Verification items for the finished model (mm, model axes). A direction names the side the tool comes from. Give positions to 0.01 mm unless a question says otherwise; leave off trailing zeros. Loops run counter-clockwise (first coordinate to the right, second up) from the corner with the lowest first, then second, coordinate; pieces in that order, holes last. Notation, with made-up numbers: (-15.75, -15.75) - (23.25, -15.75) arc R16 ccw to (23.25, 4.25) - close; hole circle Ø7 at (-31, 47.5). An arc over 180 degrees is marked (long way). One line per item, written item: value. Start each with the question number.
1. Access from +Z, -Z, +X, -X, +Y, -Y to the whole of each face (thin tool, end or side, straight path). Record for faces 1 (the cylindrical face through (-12.118, -17.56, 91.214)), 2 (the flat face through (-10, -25.292, 41)).
2. Gauge pin test, flat ends, axial feed: pin 1 (3 mm diameter, centred on y = 42, z = 33.5, fed in from +X); pin 2 (14.5 mm diameter, centred on x = 1.49, z = 55.46, fed in from -Y); pin 3 (10 mm diameter, centred on x = -9.5, z = 75, fed in from +Y); pin 4 (3 mm diameter, centred on y = 65.5, z = 53.5, fed in from +X). Record the tip position at first contact, or that the pin passes through.
3. Sectioned sample at C-C (z = 22.5). Record the cut outline in (x, y), plus the area to 3 significant figures.
4. Sectioned sample at D-D (y = 36). Record the cut outline in (x, z), plus the area to 3 significant figures.
5. Sectioned sample at B-B (y = -16.5). Count the separate pieces of the cut face and the enclosed holes in it, plus the area to 3 significant figures.
6. Sectioned sample at A-A (x = 5). Record the cut outline in (y, z).
7. Mould release check, pull along Z, two halves, no side actions. Record for faces 3 (the cylindrical face through (0.672, 35.757, 49.214)), 4 (the flat face through (-10, -25.292, 52)), 5 (the flat face through (0, 0, 100)): pulls with the +Z half, pulls with the -Z half, needs draft (parallel to the pull), parting line crosses it, or undercut.
8. Scan lines: L1, parallel to X at y = 43, z = 19.5; L2, parallel to Z at x = -0.5, y = 8; L3, parallel to Z at x = 6, y = 24. Record each from-to range of solid material in increasing order. Write a range as [from, to].
Autodesk Inventor part; units mm, degrees
ref_plane "YZ Plane" through (0, 0, 0) normal (1, 0, 0) x (0, 1, 0)
ref_plane "XZ Plane" through (0, 0, 0) normal (0, 1, 0) x (-1, 0, 0)
ref_plane "XY Plane" through (0, 0, 0) normal (0, 0, 1) x (1, 0, 0)
sketch "스케치1" plane through (0, 0, 0) normal (0, 0, 1) x (1, 0, 0)
  line L0 (-16.8705, 10.0415) -> (16.8705, 10.0415)
  line L1 (16.8705, 10.0415) -> (16.8705, -10.0415)
  line L2 (16.8705, -10.0415) -> (-16.8705, -10.0415)
  line L3 (-16.8705, -10.0415) -> (-16.8705, 10.0415)
  line L4 (-16.8705, 10.0415) -> (16.8705, -10.0415) construction
  line L5 (16.8705, 10.0415) -> (-16.8705, -10.0415) construction
  point P0 (0, 0)
extrude "돌출1" add sketch "스케치1" along normal blind 100
sketch "스케치2" plane through (-16.8705, 10.0415, 0) normal (0, 1, 0) x (1, 0, 0)
  circle A0 centre (18.3629, -19.7614) radius 11.3174
  circle A1 centre (18.3629, -55.0184) radius 11.9571
  point P0 (16.8705, 0)
extrude "돌출2" add sketch "스케치2" along normal blind 70.25
sketch "스케치3" plane through (1.4924, 80.2915, 19.7614) normal (0, 1, 0) x (1, 0, 0)
  circle A0 centre (0, 0) radius 5.7988
  circle A1 centre (0, -35.6989) radius 6.3
  point P0 (-1.4924, 19.7614)
extrude "돌출3" cut sketch "스케치3" against normal through all
sketch "스케치4" plane through (-16.8705, -10.0415, 0) normal (0, -1, 0) x (1, 0, 0)
  circle A0 centre (7.4206, 93.661) radius 3.6203
  point P0 (16.8705, 0)
extrude "돌출4" add sketch "스케치4" along normal blind 15.25
pattern_linear "직사각형 패턴1" count 9 spacing 10.5 along (0, 0, -1) of "돌출4"
sketch "스케치5" plane through (-16.8705, -10.0415, 0) normal (0, -1, 0) x (1, 0, 0)
  line L0 (27.8588, 94.265) -> (25.5194, 91.9257)
  line L1 (25.5194, 91.9257) -> (27.8178, 89.6273)
  arc A0 (27.8178, 89.6273) -> (27.8178, 91.969) centre (28.9886, 90.7982) ccw
  arc A1 (28.9886, 92.454) -> (27.8372, 93.9543) centre (29.4912, 94.0317) ccw
  arc A2 (29.6562, 92.7123) -> (28.9886, 92.454) centre (29.4017, 92.3783) ccw
  point P0 (16.8705, 0)
properties part number "0315_부품2"
Results are:
1. face 1: -Y
1. face 2: +Z, -Z, +X, -X, -Y
2. pin 1: passes through
2. pin 2: stops at y = -10.04
2. pin 3: stops at y = 10.04
2. pin 4: stops at x = 13.45
3. outline: (-16.87, -10.04) - (-12.21, -10.04) - (-12.21, -25.29) - (-6.69, -25.29) - (-6.69, -10.04) - (-3.62, -10.04) - (-3.62, 80.29) - (-9.49, 80.29) - (-9.49, 10.04) - (-16.87, 10.04) - close; (6.6, -10.04) - (16.87, -10.04) - (16.87, 10.04) - (12.47, 10.04) - (12.47, 80.29) - (6.6, 80.29) - close
3. area: 1,380 mm^2
4. outline: circle Ø23.91 at (1.49, 55.02); circle Ø22.63 at (1.49, 19.76); hole circle Ø12.6 at (1.49, 55.46); hole circle Ø11.6 at (1.49, 19.76)
4. area: 621 mm^2
5. separate pieces: 9
5. enclosed holes: 0
5. area: 371 mm^2
6. outline: (-10.04, 0) - (10.04, 0) - (10.04, 9) - (80.29, 9) - (80.29, 15.14) - (-10.04, 15.14) - close; (-10.04, 24.38) - (80.29, 24.38) - (80.29, 30.52) - (10.04, 30.52) - (10.04, 43.59) - (80.29, 43.59) - (80.29, 50.23) - (-10.04, 50.23) - close; (-10.04, 60.69) - (80.29, 60.69) - (80.29, 66.45) - (10.04, 66.45) - (10.04, 100) - (-10.04, 100) - close
7. face 3: undercut
7. face 4: needs draft
7. face 5: pulls with the +Z half
8. L1: x = [-9.82, -4.3], [7.29, 12.81]
8. L2: z = [0, 14.32], [25.21, 49.48], [61.44, 100]
8. L3: z = [9.38, 16.11], [23.41, 30.14], [43.94, 51.06], [59.86, 66.09]
